```python
from build123d import *

# Parameters (mm, degrees)
F1_DEPTH = 10
F2_R     = 5
F3_W     = 3.4494120628
F3_H     = 3.0921520665
F4_DEPTH = 25


with BuildPart() as f1:
    # F0 (on Front) → F1 (new body)
    with BuildSketch(Plane.XZ):
        with BuildLine():
            Line((9.80909843, 8.3819362969), (0.1013143445, 8.3819362969))
            ThreePointArc((0.1013143445, 8.3819362969), (1.7648005084, 6.3186167265), (3.0204653947, 3.9845688349))
            ThreePointArc((3.0204653947, 3.9845688349), (4.477852553, 2.2245980566), (5, 0))
            ThreePointArc((5, 0), (4.9706311589, -0.5411338858), (4.882869647, -1.0759107816))
            ThreePointArc((4.882869647, -1.0759107816), (6.6796718733, -2.1122029912), (8.2635629596, -3.4514896709))
            ThreePointArc((8.2635629596, -3.4514896709), (9.0582816008, -2.8412785407), (9.80909843, -2.1777957366))
            Line((9.80909843, -2.1777957366), (9.80909843, 8.3819362969))
        make_face()
        with BuildLine():
            Line((0.1013143445, 8.3819362969), (-10.19090157, 8.3819362969))
            Line((-10.19090157, 8.3819362969), (-10.19090157, -2.1777957366))
            ThreePointArc((-10.19090157, -2.1777957366), (-9.332541843, -2.9290474683), (-8.4179443125, -3.6107159674))
            ThreePointArc((-8.4179443125, -3.6107159674), (-6.7700976602, -2.1763910822), (-4.882869647, -1.0759107816))
            ThreePointArc((-4.882869647, -1.0759107816), (-2.6961548337, 4.2107896068), (3.0204653947, 3.9845688349))
            ThreePointArc((3.0204653947, 3.9845688349), (1.7648005084, 6.3186167265), (0.1013143445, 8.3819362969))
        make_face()
        with BuildLine():
            ThreePointArc((-8.4179443125, -3.6107159674), (-9.3833116946, -4.7673071134), (-10.19090157, -6.0390916293))
            Line((-10.19090157, -6.0390916293), (-10.19090157, -11.6180637031))
            Line((-10.19090157, -11.6180637031), (0.1013143445, -11.6180637031))
            ThreePointArc((0.1013143445, -11.6180637031), (2.2019143942, -8.8532431003), (3.5769410003, -5.6648178828))
            ThreePointArc((3.5769410003, -5.6648178828), (-2.6456826628, -5.9527067194), (-8.4179443125, -3.6107159674))
        make_face()
        with BuildLine():
            ThreePointArc((-4.882869647, -1.0759107816), (-6.7700976602, -2.1763910822), (-8.4179443125, -3.6107159674))
            ThreePointArc((-8.4179443125, -3.6107159674), (-2.6456826628, -5.9527067194), (3.5769410003, -5.6648178828))
            ThreePointArc((3.5769410003, -5.6648178828), (3.9117762713, -4.2721522728), (4.1061096807, -2.8530445651))
            ThreePointArc((4.1061096807, -2.8530445651), (-0.969737146, -4.9050596192), (-4.882869647, -1.0759107816))
        make_face()
        with BuildLine():
            ThreePointArc((-8.4179443125, -3.6107159674), (-9.332541843, -2.9290474683), (-10.19090157, -2.1777957366))
            Line((-10.19090157, -2.1777957366), (-10.19090157, -6.0390916293))
            ThreePointArc((-10.19090157, -6.0390916293), (-9.3833116946, -4.7673071134), (-8.4179443125, -3.6107159674))
        make_face()
        with BuildLine():
            ThreePointArc((4.1061096807, -2.8530445651), (3.9117762713, -4.2721522728), (3.5769410003, -5.6648178828))
            ThreePointArc((3.5769410003, -5.6648178828), (6.0196461638, -4.7686164468), (8.2635629596, -3.4514896709))
            ThreePointArc((8.2635629596, -3.4514896709), (6.6796718733, -2.1122029912), (4.882869647, -1.0759107816))
            ThreePointArc((4.882869647, -1.0759107816), (4.5814832161, -2.002501321), (4.1061096807, -2.8530445651))
        make_face()
        with BuildLine():
            ThreePointArc((8.2635629596, -3.4514896709), (6.0196461638, -4.7686164468), (3.5769410003, -5.6648178828))
            ThreePointArc((3.5769410003, -5.6648178828), (2.2019143942, -8.8532431003), (0.1013143445, -11.6180637031))
            Line((0.1013143445, -11.6180637031), (9.80909843, -11.6180637031))
            Line((9.80909843, -11.6180637031), (9.80909843, -5.3922310519))
            ThreePointArc((9.80909843, -5.3922310519), (9.0882832098, -4.3804872781), (8.2635629596, -3.4514896709))
        make_face()
        with BuildLine():
            Line((9.80909843, -5.3922310519), (9.80909843, -2.1777957366))
            ThreePointArc((9.80909843, -2.1777957366), (9.0582816008, -2.8412785407), (8.2635629596, -3.4514896709))
            ThreePointArc((8.2635629596, -3.4514896709), (9.0882832098, -4.3804872781), (9.80909843, -5.3922310519))
        make_face()
    extrude(amount=F1_DEPTH)

    # F2
    f2_edges = [f1.edges().sort_by_distance(p)[0] for p in [
        (9.809098, -5, 8.381936),
    ]]
    fillet(f2_edges, radius=F2_R)

    # F3 (on face) → F4 (join)
    with BuildSketch(Plane(origin=(0, 0, 0), x_dir=(-1, 0, 0), z_dir=(0, 1, 0))):
        with Locations((5.7046995498, -8.1599843688)):
            Rectangle(F3_W, F3_H)
    extrude(amount=F4_DEPTH)


solid = f1.part
```
Can you work these out from the model? Positions are in its coordinate system, mm. A direction names the side the tool comes from. Give positions to 0.01 mm unless a question says otherwise; leave off trailing zeros. Write each loop counter-clockwise with the first axis right and the second up, starting at its lowest first coordinate (ties: lowest second). Pieces come first, ordered by that corner, then holes. Notation, with made-up numbers: (-11, -34) -> (11, -34) arc R16 ccw to (11, -25) -> close; hole circle Ø10 at (4.5, 21). An arc over 180 degrees is marked (long way). Write item = value, one per line.
(1) Suppose I cut it at B-B on z = -3.75. Write out the boundary of the cut face in (x, y).
Worked out:
outline = (-10.19, -10) -> (-3.31, -10) -> (-3.31, 0) -> (-10.19, 0) -> close; (3.31, -10) -> (9.81, -10) -> (9.81, 0) -> (3.31, 0) -> close
(2) For faces 1 (the face through (-6, 12, -6.614)), 2 (the face through (-7.429, 12, -8)), 3 (the face through (-6, 12, -9.706)), which set-ups out of +Z, -Z, +X, -X, +Y, -Y let a thin tool reach every point of the face, with its end or its side?
Worked out:
face_1 = +Z, +X, -X, +Y
face_2 = +Z, -Z, -X, +Y
face_3 = -Z, +X, -X, +Y
(3) Suppose I cut it at C-C on x = -3.5. Write out the boundary of the cut face in (y, z).
Worked out:
outline = (-10, -11.62) -> (0, -11.62) -> (0, -3.57) -> (-10, -3.57) -> close; (-10, 3.57) -> (0, 3.57) -> (0, 8.38) -> (-10, 8.38) -> close
(4) I need wall thicknesses on probe 1 along X at (y, z) = (-4, -0.25); probe 2 along Y at (x, z) = (-8.75, -4.25); probe 3 along Z at (x, y) = (-4.5, 6.5). Which ranges of each line are inside material? Lowest first, please. Write a range as from..to.
Worked out:
probe_1 = -10.19..-4.99, 4.99..9.81
probe_2 = -10..0
probe_3 = -9.71..-6.61
(5) Suppose I cut it at D-D on z = -9. Write out the boundary of the cut face in (x, y).
Worked out:
outline = (-10.19, -10) -> (9.81, -10) -> (9.81, 0) -> (-3.98, 0) -> (-3.98, 25) -> (-7.43, 25) -> (-7.43, 0) -> (-10.19, 0) -> close
(6) Suppose I cut it at A-A on y = -1.5. Write out the boundary of the cut face in (x, z), then the cut area to 3 significant figures.
Worked out:
outline = (-10.19, -11.62) -> (9.81, -11.62) -> (9.81, 3.38) arc R5 ccw to (4.81, 8.38) -> (-10.19, 8.38) -> close; hole circle Ø10 at (0, 0)
area = 316 mm^2
(7) I'm going to push flat-ended pins straight in: P1, Ø1.7, axis at x = -6, y = 13, coming from the -Z side; P2, Ø3.5, axis at y = 13, z = -9, coming from the -X side; P3, Ø3, axis at x = 3.5, z = -6.5, coming from the +Y side; P4, Ø6, axis at y = 1, z = 6, coming from the +X side. Where does each tip first touch, or does it pass through?
Worked out:
P1 = -9.71
P2 = -7.43
P3 = 0
P4 = 9.81
